Here's how the part is built. I have some questions about the finished solid (model axes, mm). A direction names the side the tool comes from. Round coordinates to 2 decimals unless told otherwise and drop trailing zeros. Loops run counter-clockwise (first coordinate to the right, second up) from the corner with the lowest first, then second, coordinate; pieces in that order, holes last. Notation, with made-up numbers: M -32.75,1 L -24.75,1 A15 ccw -24.75,15 Z; hole C -33,25 d7. An arc over 180 degrees is marked long. Write each question's results on one line, items separated by ' | '. Start each with the question number.
```python
from build123d import *

# Parameters (mm, degrees)
SKETCH_1_R      = 5
EXTRUDE_1_DEPTH = 5
SKETCH_2_R      = 5
EXTRUDE_3_DEPTH = 5
EXTRUDE_4_DEPTH = 10


with BuildPart() as part:
    # Sketch 1 → Extrude 1 (new body)
    with BuildSketch(Plane(origin=(0, 0, 0), x_dir=(1, 0, 0), z_dir=(0, 1, 0))):
        with BuildLine():
            Line((20, 10), (0, 10))
            Line((0, 10), (0, -10))
            Line((0, -10), (20, -10))
            ThreePointArc((20, -10), (30, 0), (20, 10))
        make_face()
        with Locations((20, 0)):
            Circle(SKETCH_1_R, mode=Mode.SUBTRACT)
    extrude(amount=EXTRUDE_1_DEPTH)

    # Sketch 2 → Extrude 3 (add)
    with BuildSketch(Plane(origin=(0, 0, 0), x_dir=(0, 0, -1), z_dir=(1, 0, 0))):
        with BuildLine():
            Line((-10, 10), (-10, 0))
            Line((-10, 0), (10, 0))
            Line((10, 0), (10, 10))
            ThreePointArc((10, 10), (0, 20), (-10, 10))
        make_face()
        with Locations((0, 10)):
            Circle(SKETCH_2_R, mode=Mode.SUBTRACT)
    extrude(amount=EXTRUDE_3_DEPTH)

    # Sketch 2_4 → Extrude 4 (add)
    with BuildSketch(Plane(origin=(0, 0, 0), x_dir=(0, 0, -1), z_dir=(1, 0, 0))):
        Polygon((0, 5), (-10, 5), (-10, 0), (10, 0), (10, 5), align=None)
        with BuildLine():
            Line((-5, 10), (-10, 10))
            Line((-10, 10), (-10, 5))
            Line((-10, 5), (0, 5))
            ThreePointArc((0, 5), (-3.535533906, 6.464466094), (-5, 10))
        make_face()
        with BuildLine():
            Line((10, 5), (10, 10))
            Line((10, 10), (5, 10))
            ThreePointArc((5, 10), (3.535533906, 6.464466094), (0, 5))
            Line((0, 5), (10, 5))
        make_face()
    extrude(amount=EXTRUDE_4_DEPTH)


solid = part.part
```
Item 1: If we section it at A-A on x = 16: Please give me the cut outline in (y, z), and give its area (3 significant figures).
Item 2: If we section it at C-C on z = 6: Please give me the cut outline in (x, y).
Item 3: I need wall thicknesses on L1, parallel to X at y = 2.1, z = 0; L2, parallel to Z at x = 20, y = 3.2; L3, parallel to Y at x = 18.25, z = -7.5. Which ranges of each line are inside material? Lowest first, please.
Item 4: If we section it at D-D on z = 2.5: Please give me the cut outline in (x, y).
Item 5: If we section it at B-B on y = 13: Please give me the cut outline in (x, z), and give its area (3 significant figures).
Item 6: I'm going to push flat-ended pins straight in: pin 1 (10 mm diameter, centred on x = 4.5, z = 5, fed in from -Y); pin 2 (4 mm diameter, centred on x = 7.5, z = -8.5, fed in from +Y); pin 3 (1.5 mm diameter, centred on x = 22.5, z = 1.5, fed in from -Y); pin 4 (4 mm diameter, centred on x = 18, z = 8, fed in from +Y). Where does each tip first touch, or does it pass through?
Item 7: Which directions (+Z, -Z, +X, -X, +Y, -Y) give clear straight access to the entire face, cutting with the end or side of a thin tool? Please do faces 4 (the face through (8, 4, 10)), 5 (the face through (10, 8, -7)).
Item 8: If we mould it in two halves opening along X, with no side actions, what happens to faces 1 (the face through (30, 2, 0)), 2 (the face through (15, 2, 0)), 3 (the face through (15, 5, 2))? For each: released by +X, released by -X, zero draft, split by the parting line, or undercut.
Numbers:
1) outline: M 0,-10 L 5,-10 L 5,-3 L 0,-3 Z; M 0,3 L 5,3 L 5,10 L 0,10 Z | area: 70.0 mm²
2) outline: M 0,0 L 28,0 L 28,5 L 10,5 L 10,10 L 5,10 L 5,18 L 0,18 Z
3) L1: 0 to 15, 25 to 30 | L2: -10 to -5, 5 to 10 | L3: 0 to 5
4) outline: M 0,0 L 15.67,0 L 15.67,5 L 10,5 L 10,5.67 L 0,5.67 Z; M 0,14.33 L 5,14.33 L 5,19.68 L 0,19.68 Z; M 24.33,0 L 29.68,0 L 29.68,5 L 24.33,5 Z
5) outline: M 0,-9.54 L 5,-9.54 L 5,-4 L 0,-4 Z; M 0,4 L 5,4 L 5,9.54 L 0,9.54 Z | area: 55.4 mm²
6) pin 1: y = 0 | pin 2: y = 10 | pin 3: through | pin 4: y = 5
7) face 4: +Z, +X, -X, +Y, -Y | face 5: +Z, -Z, +X, +Y
8) face 1: released by +X | face 2: undercut | face 3: zero draft
